For this review, take the finished solid that the model builds, in its own axes (mm). A direction names the side the tool comes from. Give positions to 0.01 mm unless a question says otherwise; leave off trailing zeros. Use one line per item in the form item = value. Start each with the question number.
Q1. Mouldability with a two-part tool opening along X and no side actions: class faces 5 (the flat face through (35.5, 0, 2)), 6 (the flat face through (-2.5, 59, 2)), 7 (the flat face through (25, -4.6, 2)) as released by +X, released by -X, zero draft, split by the parting line, or undercut.
Q2. Tool access review of faces 1 (the flat face through (2.5, 59, 2)), 2 (the flat face through (35, -1.6, 2)), 3 (the flat face through (16, 1.5, 3)), 4 (the flat face through (30, -3, 2)): name each direction out of +Z, -Z, +X, -X, +Y, -Y from which nothing blocks a thin tool from reaching the whole face with its end or side.
Q3. Consider section A-A on z = 3. Give the number of separate pieces and of enclosed holes in the cut face, and give its area (3 significant figures).
Q4. Clearance check with flat-ended pins moving along their axes: pin 1 Ø3 at (x, z) = (22, 1.5) entering from -Y; pin 2 Ø1.5 at (x, z) = (28.5, 2) entering from -Y; pin 3 Ø0.9 at (y, z) = (-3.5, 1.5) entering from +X; pin 4 Ø0.9 at (y, z) = (59, 1.5) entering from +X. State where each tip first meets the part, or that it passes through.
Q5. For probe 1 along X at (y, z) = (58, 0.5); probe 2 along X at (y, z) = (27, 1.2); probe 3 along Y at (x, z) = (24, 3.45), list the stretches that pass through material, from the lowest coordinate up. Write a range as [from, to].
```python
from build123d import *

# Parameters (mm, degrees)
ESQUISSE3_R             = 1.863947
ESQUISSE3_R_2           = 2.023509578
ESQUISSE3_R_3           = 2.393973193
ESQUISSE3_R_4           = 1.206253728
ESQUISSE3_R_5           = 1.870132193
ESQUISSE3_R_6           = 2.067863533
ESQUISSE3_R_7           = 1.271503072
ESQUISSE3_R_8           = 1.799094092
ESQUISSE3_R_9           = 1.436016343
ESQUISSE3_R_10          = 2.031777992
ESQUISSE3_R_11          = 1.472480674
ESQUISSE3_R_12          = 1.31161039
BOSS_EXTRU_1_DEPTH      = 5
ESQUISSE4_W             = 5.690326356
ESQUISSE4_H             = 1.5
ENL_V_MAT_EXTRU_1_DEPTH = 71.522215792
CONG_1_R                = 3


with BuildPart() as part:
    # Esquisse3 → Boss.-Extru.1 (new body)
    with BuildSketch(Plane.XY):
        with BuildLine():
            Line((30, -4.6), (30, -1.6))
            Line((30, -1.6), (27, -1.6))
            Line((27, -1.6), (27, -4.6))
            Line((27, -4.6), (23, -4.6))
            Line((23, -4.6), (23, 0))
            Line((23, 0), (16, 0))
            add(Edge.make_bspline(
                [(16, 0), (-3.777040209, 10.263449678), (-7.5, 27.800800799), (-7.5, 57.73)],
                knots=[0, 0, 0, 0, 1, 1, 1, 1], degree=3))
            Line((-7.5, 57.73), (-7.5, 60.73))
            Line((-7.5, 60.73), (-2.5, 60.73))
            Line((-2.5, 60.73), (-2.5, 57.73))
            Line((-2.5, 57.73), (0, 57.73))
            Line((0, 57.73), (2.5, 57.73))
            Line((2.5, 57.73), (2.5, 60.73))
            Line((2.5, 60.73), (7.5, 60.73))
            Line((7.5, 60.73), (7.5, 57.73))
            add(Edge.make_bspline(
                [(35.5, 3.4), (-1.775512635, 10.212780912), (-5.567144123, 26.426699492), (7.5, 57.73)],
                knots=[0, 0, 0, 0, 1, 1, 1, 1], degree=3))
            Line((35.5, 3.4), (35.5, -1.6))
            Line((35.5, -1.6), (34, -1.6))
            Line((34, -1.6), (34, -4.6))
            Line((34, -4.6), (30, -4.6))
        make_face()
        with Locations((-3.815085589, 53.309291012)):
            Circle(ESQUISSE3_R, mode=Mode.SUBTRACT)
        with Locations((1.412013898, 51.930715323)):
            Circle(ESQUISSE3_R_2, mode=Mode.SUBTRACT)
        with Locations((-3.815085589, 45.669684069)):
            Circle(ESQUISSE3_R_3, mode=Mode.SUBTRACT)
        with Locations((1.412013898, 46.875937797)):
            Circle(ESQUISSE3_R_4, mode=Mode.SUBTRACT)
        with Locations((-3.010916437, 35.962213594)):
            Circle(ESQUISSE3_R_5, mode=Mode.SUBTRACT)
        with Locations((-1.804662709, 26.829149655)):
            Circle(ESQUISSE3_R_6, mode=Mode.SUBTRACT)
        with Locations((1.412013898, 16.777035258)):
            Circle(ESQUISSE3_R_7, mode=Mode.SUBTRACT)
        with Locations((8.247451688, 10.630885312)):
            Circle(ESQUISSE3_R_8, mode=Mode.SUBTRACT)
        with Locations((11.119484373, 5.461226479)):
            Circle(ESQUISSE3_R_9, mode=Mode.SUBTRACT)
        with Locations((16, 6.322836284)):
            Circle(ESQUISSE3_R_10, mode=Mode.SUBTRACT)
        with Locations((24.383722678, 3.4)):
            Circle(ESQUISSE3_R_11, mode=Mode.SUBTRACT)
        with Locations((32.413649645, 1.491605314)):
            Circle(ESQUISSE3_R_12, mode=Mode.SUBTRACT)
    extrude(amount=BOSS_EXTRU_1_DEPTH)

    # Esquisse4 → Enlèv. mat.-Extru.1 (cut, through all)
    with BuildSketch(Plane.XY.offset(5)):
        with Locations((16.154836822, 0.75)):
            Rectangle(ESQUISSE4_W, ESQUISSE4_H)
    extrude(amount=-ENL_V_MAT_EXTRU_1_DEPTH, mode=Mode.SUBTRACT)

    # Congé1
    cong_1_edges = [part.edges().sort_by_distance(p)[0] for p in [
        (35.5, 3.4, 2.5),
    ]]
    fillet(cong_1_edges, radius=CONG_1_R)


solid = part.part
```
Working result:
q1.face_5 = released by +X
q1.face_6 = undercut
q1.face_7 = zero draft
q2.face_1 = +Z, -Z, +Y
q2.face_2 = +Z, -Z, +X, -Y
q2.face_3 = +Z, -Z, -X, -Y
q2.face_4 = +Z, -Z, -Y
q3.separate_pieces = 1
q3.enclosed_holes = 12
q3.area = 546 mm²
q4.pin_1 = -4.6
q4.pin_2 = -1.6
q4.pin_3 = 34
q4.pin_4 = 7.5
q5.probe_1 = [-7.5, -2.5], [2.5, 7.5]
q5.probe_2 = [-4.82, -3.87], [0.26, 0.98]
q5.probe_3 = [-4.6, 1.98], [4.82, 6.11]
